Check sheet for the modelled part. Datum: model origin and axes. Units: mm. A direction names the side the tool comes from. Give positions to 0.01 mm unless a question says otherwise; leave off trailing zeros. Write each loop counter-clockwise with the first axis right and the second up, starting at its lowest first coordinate (ties: lowest second). Pieces come first, ordered by that corner, then holes. Notation, with made-up numbers: (-22, 48) -> (3, 48) arc R12 ccw to (3, 60) -> close; hole circle Ø1 at (33.5, 38). An arc over 180 degrees is marked (long way). Answer as a JSON object with one key per item and string values.
from build123d import *

# Parameters (mm, degrees)
SKETCH_1_R                     = 27.60110162
EXTRUDE_1_DEPTH                = 50
SPLIT_BODIES_1_SURFACE_1_BACK  = 232.061
SPLIT_BODIES_1_SURFACE_1_DEPTH = 464.122
SPLIT_BODIES_1_SURFACE_2_BACK  = 232.061
SPLIT_BODIES_1_SURFACE_2_DEPTH = 464.122


with BuildPart() as part:
    # 草图1 → 凸台-拉伸1 (new, symmetric)
    with BuildSketch(Plane.XY):
        with Locations((126.841, 106.3205)):
            Circle(SKETCH_1_R)
        with BuildLine():
            Line((0, 29.556947787), (33.841128496, 29.556947787))
            Line((33.841128496, 29.556947787), (55.404404979, 43.133825573))
            Line((55.404404979, 43.133825573), (55.404404979, 86.167316842))
            Line((55.404404979, 86.167316842), (92.202864513, 86.167316842))
            ThreePointArc((92.202864513, 86.167316842), (86.826289789, 103.279036613), (77.508707697, 118.605522617))
            ThreePointArc((77.508707697, 118.605522617), (76.622434757, 130.759815978), (87.569736188, 136.114152372))
            Line((87.569736188, 136.114152372), (152.661112554, 126.977376967))
            ThreePointArc((152.661112554, 126.977376967), (156.581939246, 124.549931981), (157.437634447, 120.018579331))
            Line((157.437634447, 120.018579331), (140.698476255, 47.962391292))
            Line((140.698476255, 47.962391292), (125.156200351, 47.962391292))
            Line((125.156200351, 47.962391292), (116.770080258, 26.493923855))
            Line((116.770080258, 26.493923855), (133.542320443, 26.493923855))
            Line((133.542320443, 26.493923855), (144.001, 0))
            Line((144.001, 0), (0, 0))
            Line((0, 0), (0, 29.556947787))
        make_face()
    extrude(amount=EXTRUDE_1_DEPTH, both=True)


with BuildPart() as body_2:
    # Split Bodies 1: the piece behind the surface
    add(part.part)
    # Split Bodies 1 surface: a surface, the sketch's curves swept straight by 464.122 mm
    with BuildLine(Plane.XY.offset(50).offset(-SPLIT_BODIES_1_SURFACE_1_BACK), mode=Mode.PRIVATE) as split_bodies_1_surface_1_path:
        Line((125.156200351, 47.962391292), (37.921543342, 47.962391292))
    split_bodies_1_surface_1 = Shell.extrude(split_bodies_1_surface_1_path.wire(), (0 * SPLIT_BODIES_1_SURFACE_1_DEPTH, 0 * SPLIT_BODIES_1_SURFACE_1_DEPTH, 1 * SPLIT_BODIES_1_SURFACE_1_DEPTH))
    split(bisect_by=split_bodies_1_surface_1, keep=Keep.BOTTOM)


with BuildPart() as part_1:
    add(part.part)

    # Split Bodies 1: split by a surface, the side it looks to stays
    # Split Bodies 1 surface: a surface, the sketch's curves swept straight by 464.122 mm
    with BuildLine(Plane.XY.offset(50).offset(-SPLIT_BODIES_1_SURFACE_2_BACK), mode=Mode.PRIVATE) as split_bodies_1_surface_2_path:
        Line((125.156200351, 47.962391292), (37.921543342, 47.962391292))
    split_bodies_1_surface_2 = Shell.extrude(split_bodies_1_surface_2_path.wire(), (0 * SPLIT_BODIES_1_SURFACE_2_DEPTH, 0 * SPLIT_BODIES_1_SURFACE_2_DEPTH, 1 * SPLIT_BODIES_1_SURFACE_2_DEPTH))
    split(bisect_by=split_bodies_1_surface_2, keep=Keep.TOP)


solid = body_2.part
1. Sectioned sample at C-C, the plane x = 120. Enter the section's corners in (y, z), plus the area to 3 significant figures.
Determined:
{"outline": "(47.96, -50) -> (133.06, -50) -> (133.06, 50) -> (47.96, 50) -> close", "area": "8,510 mm^2"}
2. Scan lines: L1, parallel to Y at x = 68, z = 7.5; L2, parallel to Y at x = 77.5, z = 38; L3, parallel to Y at x = 84, z = 9. Record each from-to range of solid material in increasing order. Write a range as [from, to].
Determined:
{"L1": "[47.96, 86.17]", "L2": "[47.96, 86.17], [118.62, 132.06]", "L3": "[47.96, 86.17], [108.88, 136.02]"}
3. Go/stop test with flat-tipped pins: P1, Ø11, axis at x = 65, z = -2, coming from the +Y side; P2, Ø1.5, axis at x = 136, z = -13.5, coming from the +Y side; P3, Ø1, axis at x = 114, z = 38.5, coming from the +Y side. Record where each tip stops, or that it passes through.
Determined:
{"P1": "y = 86.17", "P2": "y = 132.61", "P3": "y = 132.47"}
4. Access from +Z, -Z, +X, -X, +Y, -Y to the whole of each face (thin tool, end or side, straight path). Record for faces 4 (the face through (101.962, 134.094, 0.7)), 5 (the face through (106, 93, 50)), 6 (the face through (86.93, 103.05, 0.7)).
Determined:
{"face 4": "+Z, -Z, +Y", "face 5": "+Z, +X, -X, +Y, -Y", "face 6": "+Z, -Z, -X"}
5. Sectioned sample at B-B, the plane y = 99. Enter the section's corners in (x, z).
Determined:
{"outline": "(88.61, -50) -> (153.45, -50) -> (153.45, 50) -> (88.61, 50) -> close"}
6. Mould release check, pull along Y, two halves, no side actions. Record for faces 1 (the face through (74, 86.167, 1)), 2 (the face through (148.07, 127.62, 0.7)), 3 (the face through (55.404, 67, 1)): released by +Y, released by -Y, zero draft, split by the parting line, or undercut.
Determined:
{"face 1": "undercut", "face 2": "released by +Y", "face 3": "zero draft"}
7. Sectioned sample at A-A, the plane z = -35. Enter the section's corners in (x, y), plus the area to 3 significant figures.
Determined:
{"outline": "(55.4, 47.96) -> (140.7, 47.96) -> (151.27, 93.48) arc R27.6 ccw to (154.43, 107.08) -> (157.44, 120.02) arc R5.72 ccw to (152.66, 126.98) -> (143.6, 128.25) arc R27.6 ccw to (116.76, 132.02) -> (87.57, 136.11) arc R10.88 ccw to (77.51, 118.61) arc R74.36 cw to (92.2, 86.17) -> (55.4, 86.17) -> close", "area": "6,740 mm^2"}
